from build123d import *

# Parameters (mm, degrees)
F0_W     = 97.43362
F0_H     = 72.795242
F1_DEPTH = 50.8
F2_R     = 15.875
F3_DEPTH = 72.796242


with BuildPart() as f1:
    # F0 (on Top) → F1 (new body)
    with BuildSketch(Plane.XY):
        Rectangle(F0_W, F0_H)
    extrude(amount=F1_DEPTH)

    # F2 (on face) → F3 (cut, through all)
    with BuildSketch(Plane.XZ.offset(36.397621)):
        with Locations((-19.05, 50.8)):
            Circle(F2_R)
        with Locations((19.05, 50.8)):
            Circle(F2_R)
    extrude(amount=-F3_DEPTH, mode=Mode.SUBTRACT)


solid = f1.part
The model under review builds one solid part; all positions refer to its coordinate system, in mm. Coordinates: 2 decimals unless noted, no trailing zeros. Loops run counter-clockwise (first coordinate to the right, second up) from the corner with the lowest first, then second, coordinate; pieces in that order, holes last.
(1) Consider section C-C, the plane x = -25. Give the boundary of the cut face in (y, z), plus the area to 3 significant figures.
Determined:
outline: (-36.4, 0) - (36.4, 0) - (36.4, 36.08) - (-36.4, 36.08) - close
area: 2,630 mm2
(2) Wall thickness on L1, parallel to X at y = 18, z = 46.5; L2, parallel to X at y = 21, z = 45; L3, parallel to Z at x = -5.5, y = -24.5: over which ranges is each line inside the solid? List them lowest first.
Determined:
L1: x = -48.72 to -34.33, -3.77 to 3.77, 34.33 to 48.72
L2: x = -48.72 to -33.83, -4.27 to 4.27, 33.83 to 48.72
L3: z = 0 to 42.53
(3) Insertion check: P1, Ø12, axis at x = -18, z = 45, coming from the +Y side; P2, Ø4, axis at x = -18.5, y = -22, coming from the +Z side. Each pin has a flat end and moves straight along its axis. Give the tip position at first contact, or say it passes through.
Determined:
P1: passes through
P2: stops at z = 35.13
(4) Consider section B-B, the plane y = 11. Give the boundary of the cut face in (x, z) (3 decimals).
Determined:
outline: (-48.717, 0) - (48.717, 0) - (48.717, 50.8) - (34.925, 50.8) arc R15.875 cw to (3.175, 50.8) - (-3.175, 50.8) arc R15.875 cw to (-34.925, 50.8) - (-48.717, 50.8) - close
(5) Consider section D-D, the plane x = 5. Give the boundary of the cut face in (y, z).
Determined:
outline: (-36.4, 0) - (36.4, 0) - (36.4, 43.41) - (-36.4, 43.41) - close
(6) Draft analysis for pull direction X (two halves, no side actions). For faces 1 (the flat face through (-48.717, -1, 25)), 2 (the cylindrical face through (18.7, -0.51, 34.93)), 3 (the flat face through (-42, 1, 50.8)), state which applies: +X half, -X half, draft (parallel to the pull), parting line (faces both ways), or undercut.
Determined:
face 1: -X half
face 2: undercut
face 3: draft
(7) Consider section A-A, the plane z = 42. Give the boundary of the cut face in (x, y).
Determined:
outline: (-48.72, -36.4) - (-32.26, -36.4) - (-32.26, 36.4) - (-48.72, 36.4) - close; (-5.84, -36.4) - (5.84, -36.4) - (5.84, 36.4) - (-5.84, 36.4) - close; (32.26, -36.4) - (48.72, -36.4) - (48.72, 36.4) - (32.26, 36.4) - close
